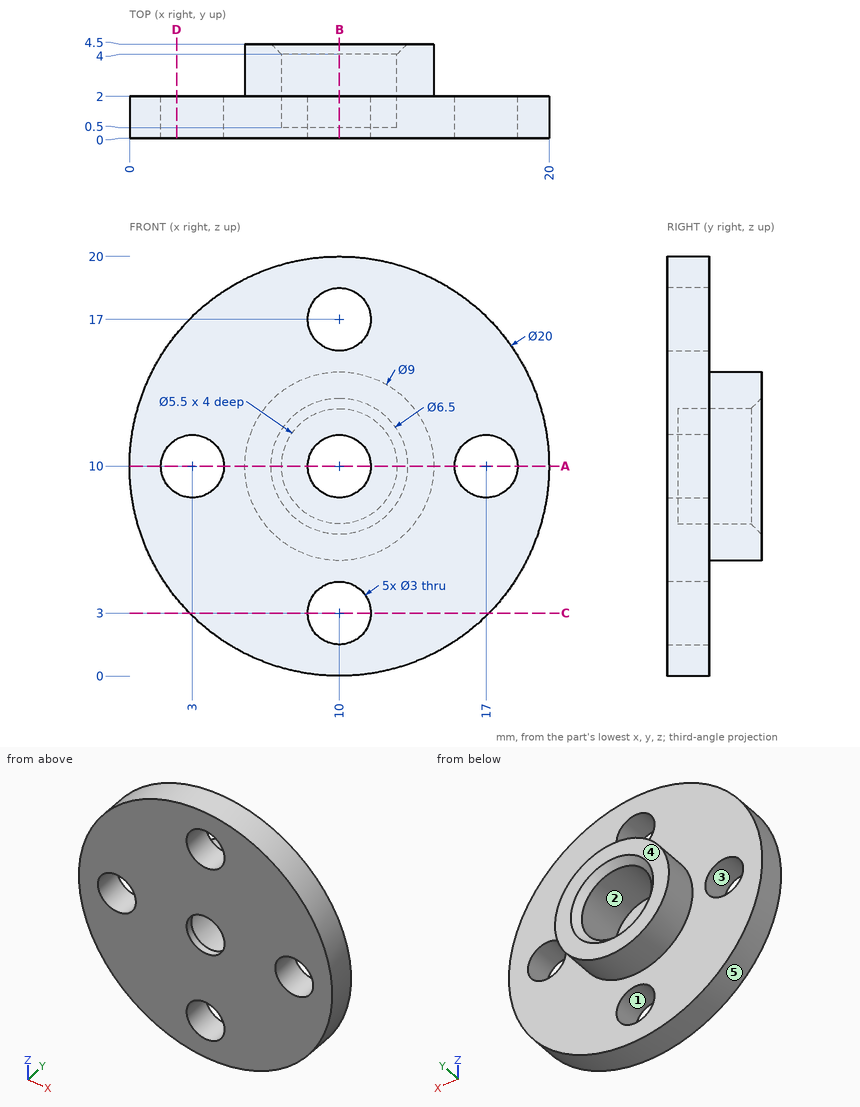
Source: three-view drawing plus pictorial views. Frame: mm from the lowest corner of the part. A direction names the side the tool comes from. Round coordinates to 2 decimals unless told otherwise and drop trailing zeros. Write each loop counter-clockwise with the first axis right and the second up, starting at its lowest first coordinate (ties: lowest second). Pieces come first, ordered by that corner, then holes. Notation, with made-up numbers: M 59.25,64 L 97.25,64 A37 ccw 97.25,103 Z; hole C 83,79.5 d8. An arc over 180 degrees is marked long. One line per item, written item: value. Start each with the question number.
Item 1: Set-up query: the marked faces 1 and 2. Return all of +Z, -Z, +X, -X, +Y, -Y with unobstructed straight access to the full face (end or side cutting, diameter ignored); none if empty.
Item 2: Pin query (flat end, axial travel): pin 1 (3.5 mm diameter, centred on x = 10, z = 10, fed in from +Y); pin 2 (1.5 mm diameter, centred on y = 2.5, z = 13, fed in from +X); pin 3 (3.5 mm diameter, centred on x = 10, z = 17, fed in from +Y). Return the tip coordinate at first contact, or that it passes through.
Item 3: Section query C-C (z = 3). Return the cut outline in (x, y), plus the area to 3 significant figures.
Item 4: Section query D-D (x = 2.25). Return the cut outline in (y, z), plus the area to 3 significant figures.
Item 5: Mould query, pull axis X, two halves, no side actions, for the marked faces 3, 4 and 5. Classes: pulls with the +X half, pulls with the -X half, needs draft (parallel to the pull), parting line crosses it, or undercut.
Item 6: Section query A-A (z = 10). Return the cut outline in (x, y).
Item 7: Section query B-B (x = 10). Return the cut outline in (y, z).
Item 8: Ray query, L1, parallel to X at y = 1.25, z = 10; L2, parallel to X at y = 0.25, z = 10; L3, parallel to X at y = 2.85, z = 10. Return the intervals inside material, ascending. Write a range as from..to.
Result set:
1. face 1: +Y, -Y
1. face 2: +Y
2. pin 1: stops at y = 0.5
2. pin 2: stops at x = 19.7
2. pin 3: stops at y = 2
3. outline: M 2.86,0 L 8.5,0 L 8.5,2 L 2.86,2 Z; M 11.5,0 L 17.14,0 L 17.14,2 L 11.5,2 Z
3. area: 22.6 mm²
4. outline: M 0,3.68 L 2,3.68 L 2,8.7 L 0,8.7 Z; M 0,11.3 L 2,11.3 L 2,16.32 L 0,16.32 Z
4. area: 20.1 mm²
5. face 3: undercut
5. face 4: needs draft
5. face 5: parting line crosses it
6. outline: M 0,0 L 1.5,0 L 1.5,2 L 0,2 Z; M 4.5,0 L 8.5,0 L 8.5,0.5 L 7.25,0.5 L 7.25,4 L 6.75,4.5 L 5.5,4.5 L 5.5,2 L 4.5,2 Z; M 11.5,0 L 15.5,0 L 15.5,2 L 14.5,2 L 14.5,4.5 L 13.25,4.5 L 12.75,4 L 12.75,0.5 L 11.5,0.5 Z; M 18.5,0 L 20,0 L 20,2 L 18.5,2 Z
7. outline: M 0,0 L 2,0 L 2,1.5 L 0,1.5 Z; M 0,4.5 L 2,4.5 L 2,5.5 L 4.5,5.5 L 4.5,6.75 L 4,7.25 L 0.5,7.25 L 0.5,8.5 L 0,8.5 Z; M 0,11.5 L 0.5,11.5 L 0.5,12.75 L 4,12.75 L 4.5,13.25 L 4.5,14.5 L 2,14.5 L 2,15.5 L 0,15.5 Z; M 0,18.5 L 2,18.5 L 2,20 L 0,20 Z
8. L1: x = 0..1.5, 4.5..7.25, 12.75..15.5, 18.5..20
8. L2: x = 0..1.5, 4.5..8.5, 11.5..15.5, 18.5..20
8. L3: x = 5.5..7.25, 12.75..14.5
